from build123d import *

# Parameters (mm, degrees)
BOSS_EXTRUDE1_DEPTH = 40
SKETCH2_R           = 2
BOSS_EXTRUDE2_DEPTH = 317
SKETCH3_W           = 461.580426742
SKETCH3_H           = 331.625976184
BOSS_EXTRUDE3_DEPTH = 4


with BuildPart() as part:
    # Sketch1 → Boss-Extrude1 (new body)
    with BuildSketch(Plane(origin=(0, 0, 0), x_dir=(1, 0, 0), z_dir=(0, 1, 0))):
        Polygon((-37.739281915, 72.174102179), (-143.805299093, 178.240119357), (-299.368790954, 333.803611218), (-319.365770726, 313.806631446), (-163.802279668, 158.243140388), (-57.739282705, 52.174103081), (-57.739282705, -52.174103272), (-163.80227984, -158.243140407), (-319.361342305, -313.811061538), (-299.36379317, -333.807471931), (-143.805300025, -178.240120135), (-37.739282847, -72.174102957), (37.739282893, -72.174102957), (143.805300071, -178.240120135), (299.368791932, -333.803611997), (319.365771704, -313.806632225), (163.802280352, -158.243140872), (57.739283379, -52.174103575), (57.739283379, 52.174102471), (163.802280509, 158.243139611), (319.361342965, 313.811060751), (299.36379383, 333.807471143), (143.805300678, 178.240119357), (37.7392835, 72.174102179), align=None)
    extrude(amount=BOSS_EXTRUDE1_DEPTH)

    # Sketch2 → Boss-Extrude2 (add)
    with BuildSketch(Plane(origin=(0, 0, 0), x_dir=(-1, 0, 0), z_dir=(0, -1, 0))):
        with Locations(Location((0, 0, 0), (0, 0, 90))):
            Circle(SKETCH2_R)
    extrude(amount=BOSS_EXTRUDE2_DEPTH)

    # Sketch3 → Boss-Extrude3 (add)
    with BuildSketch(Plane.XZ.offset(317)):
        Rectangle(SKETCH3_W, SKETCH3_H)
    extrude(amount=BOSS_EXTRUDE3_DEPTH)


solid = part.part
Source: CAD feature listing. Evaluate the final solid. Frame: model axes, mm. A direction names the side the tool comes from. Coordinates: 2 decimals unless noted, no trailing zeros. Loops run counter-clockwise (first coordinate to the right, second up) from the corner with the lowest first, then second, coordinate; pieces in that order, holes last. Notation, with made-up numbers: (40.25, -20.5) -> (69.25, -20.5) arc R6 ccw to (69.25, -16.5) -> close; hole circle Ø4 at (13.5, -29.5). An arc over 180 degrees is marked (long way). Answer in a Markdown table with one row per item. Add a question column.
Q1. Section B-B on x = 92. Return the cut outline in (y, z), and give its area (3 significant figures).
Q2. Pull-direction query (X, two-part tool) for faces 4 (the face through (57.739, 20, 1)), 5 (the face through (-309.227, 19.72, -323.945)), 6 (the face through (-3, -317, 2)), 7 (the face through (-1, 20, 72.174)); classes: pulls with the +X half, pulls with the -X half, needs draft (parallel to the pull), parting line crosses it, or undercut.
Q3. Section A-A on z = -42. Return the cut outline in (x, y), and give its area (3 significant figures).
Q4. Section D-D on y = -262.5. Return the cut outline in (x, z), and give its area (3 significant figures).
Q5. Contact query for flat-ended pins moving along their axis: pin 1 Ø3 at (y, z) = (-318, -82.5) entering from -X; pin 2 Ø8 at (x, y) = (100, 1.5) entering from -Z; pin 3 Ø3 at (x, y) = (112, -319.5) entering from +Z. Output: stop coordinate, or through.
Q6. Ray query, line 1 along Y through (x, z) = (152.5, -115); line 2 along Y through (x, z) = (249, 254.5). Return the intervals inside material, ascending.
Q7. Section C-C on x = -254. Return the cut outline in (y, z), and give its area (3 significant figures).
Q8. Reachability of faces 1 (the face through (-166.723, 19.72, -201.157)), 2 (the face through (-309.5, 19.72, 323.67)), 3 (the face through (-57.739, 20, -1)) from +Z, -Z, +X, -X, +Y, -Y: full face, straight path, thin tool, end or side. Return the list, or none.
Computed values:
| question | item | result |
|---|---|---|
| 1 | outline | (-321, -165.81) -> (-317, -165.81) -> (-317, 165.81) -> (-321, 165.81) -> close; (0, -126.43) -> (40, -126.43) -> (40, -86.44) -> (0, -86.44) -> close; (0, 86.44) -> (40, 86.44) -> (40, 126.43) -> (0, 126.43) -> close |
| 1 | area | 4,530 mm^2 |
| 2 | face 4 | pulls with the +X half |
| 2 | face 5 | pulls with the -X half |
| 2 | face 6 | needs draft |
| 2 | face 7 | undercut |
| 3 | outline | (-230.79, -321) -> (230.79, -321) -> (230.79, -317) -> (-230.79, -317) -> close; (-57.74, 0) -> (57.74, 0) -> (57.74, 40) -> (-57.74, 40) -> close |
| 3 | area | 6,470 mm^2 |
| 4 | outline | circle Ø4 at (0, 0) |
| 4 | area | 12.6 mm^2 |
| 5 | pin 1 | stops at x = -230.79 |
| 5 | pin 2 | stops at z = -138.43 |
| 5 | pin 3 | stops at z = 165.81 |
| 6 | line 1 | y = -321 to -317 |
| 6 | line 2 | y = 0 to 40 |
| 7 | outline | (0, -288.43) -> (40, -288.43) -> (40, -248.44) -> (0, -248.44) -> close; (0, 248.45) -> (40, 248.45) -> (40, 288.44) -> (0, 288.44) -> close |
| 7 | area | 3,200 mm^2 |
| 8 | face 1 | -Z, +Y |
| 8 | face 2 | +Z, -X, +Y, -Y |
| 8 | face 3 | -X, +Y |
